Here's how the part is built. I have some questions about the finished solid (model axes, mm). Face numbers are marked on the shaded views. A direction names the side the tool comes from. Round coordinates to 2 decimals unless told otherwise and drop trailing zeros. Loops run counter-clockwise (first coordinate to the right, second up) from the corner with the lowest first, then second, coordinate; pieces in that order, holes last. Notation, with made-up numbers: (-15.75, -31.5) -> (20.25, -31.5) arc R14 cw to (20.25, -14.5) -> close; hole circle Ø9 at (-27, 32.25). An arc over 180 degrees is marked (long way). Use one line per item in the form item = value. Start each with the question number.
Item 1: For the marked faces 1, 2 and 3, which set-ups out of +Z, -Z, +X, -X, +Y, -Y let a thin tool reach every point of the face, with its end or its side?
Item 2: Thinking about a two-plate mould opening in Y: for the marked faces 4, 5 and 6, which applies, released by +Y, released by -Y, zero draft, split by the parting line, or undercut?
Item 3: I'm going to push flat-ended pins straight in: pin 1 Ø5 at (y, z) = (0.5, 10) entering from -X; pin 2 Ø1.5 at (y, z) = (-5, 2) entering from +X; pin 3 Ø2 at (x, z) = (-3.5, 0.5) entering from -Y; pin 4 Ø5.5 at (x, z) = (10.5, 10.5) entering from -Y. Where does each tip first touch, or does it pass through?
Item 4: If I drill on L1, parallel to Z at x = 14.6, y = 0; L2, parallel to Y at x = 0, z = -1.5; L3, parallel to X at y = -2, z = 11.25, over which ranges is the centre line in solid material (lowest first)? Write a range as [from, to].
Item 5: If we section it at B-B (x = 0): Write out the boundary of the cut face in (y, z), then the cut area to 4 significant figures.
Item 6: If we section it at A-A (z = 13.5): Write out the boundary of the cut face in (x, y), then the cut area to 3 significant figures.
Item 7: If we section it at D-D (y = -5): Write out the boundary of the cut face in (x, z), then the cut area to 3 significant figures.
Item 8: If we section it at C-C (z = 11): Write out the boundary of the cut face in (x, y).
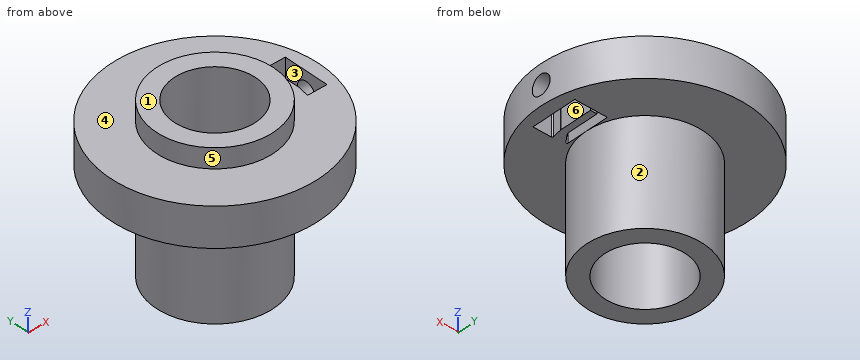
```python
from build123d import *

# Parameters (mm, degrees)
SKIZZE1_R                       = 9
SKIZZE1_R_2                     = 6.25
AUFSATZ_LINEAR_AUSTRAGEN1_DEPTH = 8
SKIZZE2_R                       = 16
SKIZZE2_R_2                     = 6.25
AUFSATZ_LINEAR_AUSTRAGEN2_DEPTH = 6
SCHNITT_LINEAR_AUSTRAGEN1_DEPTH = 6
SCHNITT_LINEAR_START            = 17
SKIZZE4_R                       = 1.5
SCHNITT_LINEAR_AUSTRAGEN2_DEPTH = 4
SKIZZE5_R                       = 9
SKIZZE5_R_2                     = 6.25
AUFSATZ_LINEAR_AUSTRAGEN3_DEPTH = 3
VERRUNDUNG1_R                   = 0.15
VERRUNDUNG2_R                   = 0.15


with BuildPart() as part:
    # Skizze1 → Aufsatz-Linear austragen1 (new, symmetric)
    with BuildSketch(Plane.XY):
        Circle(SKIZZE1_R)
        Circle(SKIZZE1_R_2, mode=Mode.SUBTRACT)
    extrude(amount=AUFSATZ_LINEAR_AUSTRAGEN1_DEPTH, both=True)

    # Skizze2 → Aufsatz-Linear austragen2 (add)
    with BuildSketch(Plane.XY.offset(8)):
        Circle(SKIZZE2_R)
        Circle(SKIZZE2_R_2, mode=Mode.SUBTRACT)
    extrude(amount=AUFSATZ_LINEAR_AUSTRAGEN2_DEPTH)

    # Skizze3 → Schnitt-Linear austragen1 (cut)
    with BuildSketch(Plane(origin=(0, 0, 8), x_dir=(-1, 0, 0), z_dir=(0, 0, -1))):
        with BuildLine():
            Line((-9, -3.5), (-10.094357833, -2.06891668))
            ThreePointArc((-10.094357833, -2.06891668), (-10.24719529, -1.78212384), (-10.3, -1.461466572))
            Line((-10.3, -1.461466572), (-10.3, 3.2))
            Line((-10.3, 3.2), (-11.3, 3.2))
            Line((-11.3, 3.2), (-11.3, -1.712441166))
            ThreePointArc((-11.3, -1.712441166), (-11.296188626, -1.799666281), (-11.284783559, -1.8862265))
            Line((-11.284783559, -1.8862265), (-11, -3.5))
            Line((-11, -3.5), (-14, -3.5))
            Line((-14, -3.5), (-14, 3.5))
            Line((-14, 3.5), (-9, 3.5))
            Line((-9, 3.5), (-9, -3.5))
        make_face()
    extrude(amount=-SCHNITT_LINEAR_AUSTRAGEN1_DEPTH, mode=Mode.SUBTRACT)

    # Skizze4 → Schnitt-Linear austragen2 (cut)
    with BuildSketch(Plane(origin=(0, 0, 0), x_dir=(0, 0, -1), z_dir=(1, 0, 0)).offset(SCHNITT_LINEAR_START)):
        with Locations((-11, 0)):
            Circle(SKIZZE4_R)
    extrude(amount=-SCHNITT_LINEAR_AUSTRAGEN2_DEPTH, mode=Mode.SUBTRACT)

    # Skizze5 → Aufsatz-Linear austragen3 (add)
    with BuildSketch(Plane.XY.offset(14)):
        Circle(SKIZZE5_R)
        Circle(SKIZZE5_R_2, mode=Mode.SUBTRACT)
    extrude(amount=AUFSATZ_LINEAR_AUSTRAGEN3_DEPTH)

    # Verrundung1
    verrundung1_edges = [part.edges().sort_by_distance(p)[0] for p in [
        (9, -3.5, 11),
    ]]
    fillet(verrundung1_edges, radius=VERRUNDUNG1_R)

    # Verrundung2
    verrundung2_edges = [part.edges().sort_by_distance(p)[0] for p in [
        (11, -3.5, 11),
    ]]
    fillet(verrundung2_edges, radius=VERRUNDUNG2_R)


solid = part.part
```
Values found:
q1.face_1 = +Z, +X, -X, +Y, -Y
q1.face_2 = -Z
q1.face_3 = +Z, -Z
q2.face_4 = zero draft
q2.face_5 = split by the parting line
q2.face_6 = undercut
q3.pin_1 = -16
q3.pin_2 = 7.93
q3.pin_3 = -8.65
q3.pin_4 = -14
q4.L1 = [8, 9.5], [12.5, 14]
q4.L2 = [-9, -6.25], [6.25, 9]
q4.L3 = [-15.87, -5.92], [5.92, 9], [10.14, 11.26], [14, 15.87]
q5.outline = (-16, 8) -> (-9, 8) -> (-9, -8) -> (-6.25, -8) -> (-6.25, 17) -> (-9, 17) -> (-9, 14) -> (-16, 14) -> close; (6.25, -8) -> (9, -8) -> (9, 8) -> (16, 8) -> (16, 14) -> (9, 14) -> (9, 17) -> (6.25, 17) -> close
q5.area = 221.5 mm2
q6.outline = circle Ø32 at (0, 0); hole circle Ø12.5 at (0, 0); hole (9, -3.06) arc R0.15 ccw to (9.27, -3.15) -> (10.09, -2.07) arc R1 ccw to (10.3, -1.46) -> (10.3, 3.2) -> (11.3, 3.2) -> (11.3, -1.71) arc R1 cw to (11.28, -1.89) -> (11.03, -3.32) arc R0.15 ccw to (11.18, -3.5) -> (14, -3.5) -> (14, 3.5) -> (9, 3.5) -> close
q6.area = 654 mm2
q7.outline = (-15.2, 8) -> (-7.48, 8) -> (-7.48, -8) -> (-3.75, -8) -> (-3.75, 17) -> (-7.48, 17) -> (-7.48, 14) -> (-15.2, 14) -> close; (3.75, -8) -> (7.48, -8) -> (7.48, 8) -> (15.2, 8) -> (15.2, 14) -> (7.48, 14) -> (7.48, 17) -> (3.75, 17) -> close
q7.area = 279 mm2
q8.outline = (9, -3.06) -> (9, 3.5) -> (14, 3.5) -> (14, 1.5) -> (15.93, 1.5) arc R16 ccw (long way) to (15.93, -1.5) -> (14, -1.5) -> (14, -3.5) -> (11.18, -3.5) arc R0.15 cw to (11.03, -3.32) -> (11.28, -1.89) arc R1 ccw to (11.3, -1.71) -> (11.3, 3.2) -> (10.3, 3.2) -> (10.3, -1.46) arc R1 cw to (10.09, -2.07) -> (9.27, -3.15) arc R0.15 cw to start; hole circle Ø12.5 at (0, 0)
